Source: three-view drawing plus pictorial views. Frame: mm from the lowest corner of the part. A direction names the side the tool comes from. Round coordinates to 2 decimals unless told otherwise and drop trailing zeros. Write each loop counter-clockwise with the first axis right and the second up, starting at its lowest first coordinate (ties: lowest second). Pieces come first, ordered by that corner, then holes. Notation, with made-up numbers: M 12.5,72.25 L 31.5,72.25 A30 cw 31.5,96.25 Z; hole C -9.75,22 d1. An arc over 180 degrees is marked long. Put each result on its own line as item: value. Start each with the question number.
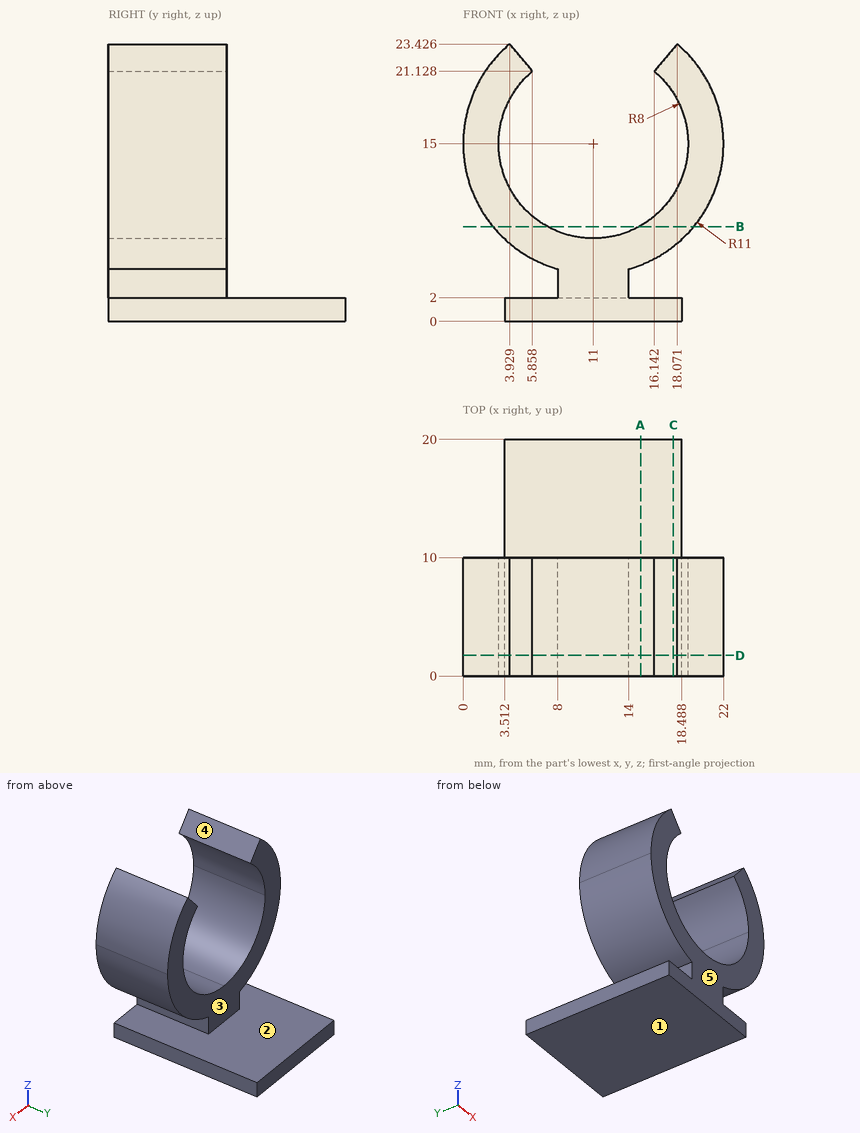
(1) Section query B-B (z = 8). Return loops of the section in (x, y) (1 decimal).
(2) Ray query, line 1 along X through (y, z) = (4.5, 4.25); line 2 along Y through (x, z) = (3.5, 10.25); line 3 along Z through (x, y) = (17, 10.25). Return the intervals inside material, ascending.
(3) Contact query for flat-ended pins moving along their axis: P1, Ø10.5, axis at x = 11.5, z = 7.5, coming from the +Y side; P2, Ø1.2, axis at y = 2.5, z = 3, coming from the +X side; P3, Ø12, axis at x = 10.5, y = 6, coming from the +Z side (1 decimal). Output: stop coordinate, or through.
(4) Access query for the marked faces 4 and 5. Directions: +Z, -Z, +X, -X, +Y, -Y. A direction counts if a zero-diameter tool reaches every point of the face in a straight line with its end or side. Return the directions, or none.
(5) Section query D-D (y = 1.75). Return loops of the section in (x, z), and give its area (3 significant figures).
(6) Section query A-A (x = 15). Return loops of the section in (y, z).
(7) Section query C-C (x = 17.75). Return loops of the section in (y, z) (1 decimal).
(8) Pull-direction query (Z, two-part tool) for the marked faces 1, 2 and 3; classes: +Z half, -Z half, draft (parallel to the pull), parting line (faces both ways), or undercut.
Entries:
1. outline: M 2.5,0 L 7.1,0 L 7.1,10 L 2.5,10 Z; M 14.9,0 L 19.5,0 L 19.5,10 L 14.9,10 Z
2. line 1: 8 to 14
2. line 2: 0 to 10
2. line 3: 0 to 2
3. P1: y = 10
3. P2: x = 14
3. P3: z = 22.7
4. face 4: +Z, +Y, -Y
4. face 5: +Z, -Z, +X, -X, -Y
5. outline: M 3.51,0 L 18.49,0 L 18.49,2 L 14,2 L 14,4.42 A11 ccw 18.07,23.43 L 16.14,21.13 A8 cw long 5.86,21.13 L 3.93,23.43 A11 ccw 8,4.42 L 8,2 L 3.51,2 Z
5. area: 182 mm2
6. outline: M 0,0 L 20,0 L 20,2 L 0,2 Z; M 0,4.75 L 10,4.75 L 10,8.07 L 0,8.07 Z
7. outline: M 0,0 L 20,0 L 20,2 L 0,2 Z; M 0,6.3 L 10,6.3 L 10,10.7 L 0,10.7 Z; M 0,19.3 L 10,19.3 L 10,23 L 0,23 Z
8. face 1: -Z half
8. face 2: undercut
8. face 3: draft
